The drawing under review shows one solid part. Ordinate dimensions are in mm from its lowest x, y, z. A direction names the side the tool comes from. Coordinates: 2 decimals unless noted, no trailing zeros. Write each loop counter-clockwise with the first axis right and the second up, starting at its lowest first coordinate (ties: lowest second). Pieces come first, ordered by that corner, then holes. Notation, with made-up numbers: M 30.5,-29.5 L 50.5,-29.5 A16 ccw 50.5,-4.5 Z; hole C -38,-20.75 d2. An arc over 180 degrees is marked long. Write item = value, one per line.
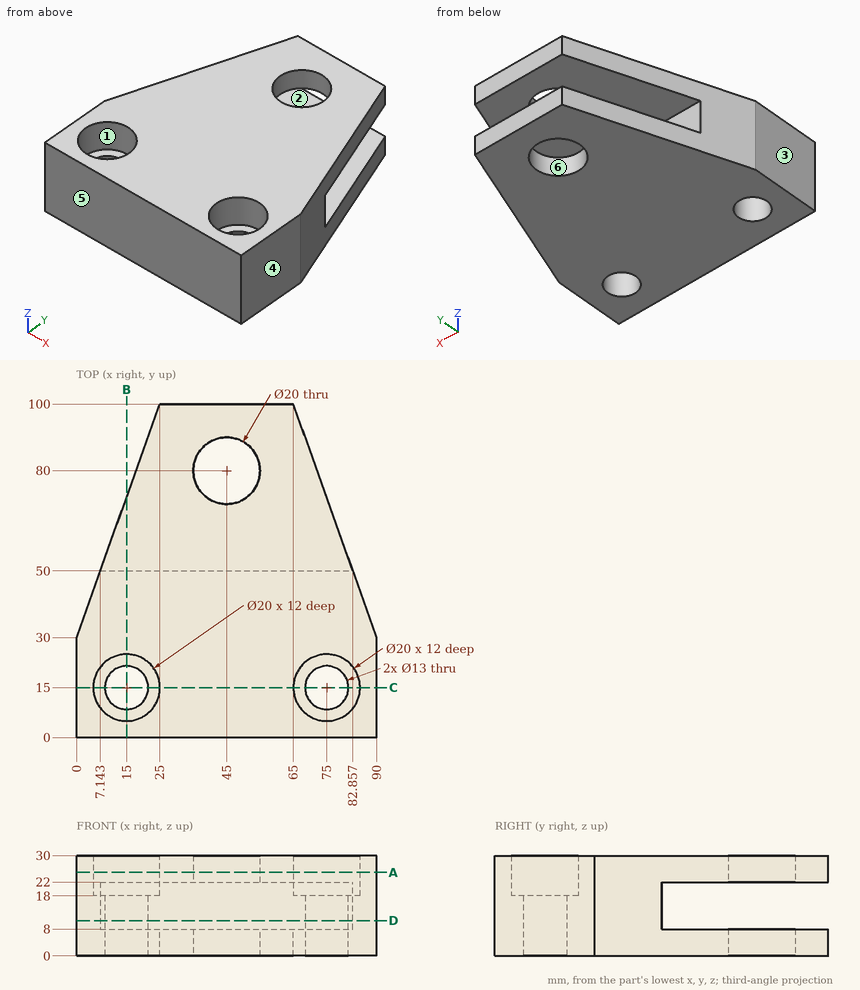
Q1. Consider section C-C, the plane y = 15. State the section outline as (x, z) points, and give its area (3 significant figures).
Check result:
outline = M 0,0 L 8.5,0 L 8.5,18 L 5,18 L 5,30 L 0,30 Z; M 21.5,0 L 68.5,0 L 68.5,18 L 65,18 L 65,30 L 25,30 L 25,18 L 21.5,18 Z; M 81.5,0 L 90,0 L 90,30 L 85,30 L 85,18 L 81.5,18 Z
area = 1,750 mm²
Q2. For P1, Ø16, axis at x = 75, y = 15, coming from the +Z side; P2, Ø16, axis at x = 45, y = 80, coming from the +Z side; P3, Ø2, axis at x = 17, z = 19, coming from the +Y side, all flat-tipped, find the tip position at first contact; note any pin that passes through.
Check result:
P1 = 18
P2 = through
P3 = 50
Q3. Consider section B-B, the plane x = 15. State the section outline as (y, z) points.
Check result:
outline = M 0,0 L 8.5,0 L 8.5,18 L 5,18 L 5,30 L 0,30 Z; M 21.5,0 L 72,0 L 72,8 L 50,8 L 50,22 L 72,22 L 72,30 L 25,30 L 25,18 L 21.5,18 Z
Q4. Machinability: for the marked faces 1, 2 and 3, which of the approach directions +Z, -Z, +X, -X, +Y, -Y give a long, thin tool a straight path to every point of the face, cutting with its end or side? Answer none if there is none.
Check result:
face_1 = +Z
face_2 = +X, -X, +Y
face_3 = +Z, -Z, -X, +Y, -Y
Q5. Consider section D-D, the plane z = 10.5. State the section outline as (x, y) points, and give its area (3 significant figures).
Check result:
outline = M 0,0 L 90,0 L 90,30 L 82.86,50 L 7.14,50 L 0,30 Z; hole C 15,15 d13; hole C 75,15 d13
area = 4,090 mm²
Q6. The part is to be moulded in two halves that separate along X. For the marked faces 4, 5 and 6, say which applies: +X half, -X half, draft (parallel to the pull), parting line (faces both ways), or undercut.
Check result:
face_4 = +X half
face_5 = draft
face_6 = undercut
Q7. Consider section A-A, the plane z = 25. State the section outline as (x, y) points, and give its area (3 significant figures).
Check result:
outline = M 0,0 L 90,0 L 90,30 L 65,100 L 25,100 L 0,30 Z; hole C 15,15 d20; hole C 45,80 d20; hole C 75,15 d20
area = 6,310 mm²
Q8. Wall thickness on line 1 (Y direction, x = 45, z = 25.25); line 2 (Z direction, x = 27.5, y = 87); line 3 (Y direction, x = 75, z = 12): over which ranges is each line inside the solid? List them lowest first.
Check result:
line_1 = 0 to 70, 90 to 100
line_2 = 0 to 8, 22 to 30
line_3 = 0 to 8.5, 21.5 to 50
